Here's how the part is built. I have some questions about the finished solid (model axes, mm). Face numbers are marked on the shaded views. A direction names the side the tool comes from. Coordinates: 2 decimals unless noted, no trailing zeros. Write each loop counter-clockwise with the first axis right and the second up, starting at its lowest first coordinate (ties: lowest second). Pieces come first, ordered by that corner, then holes.
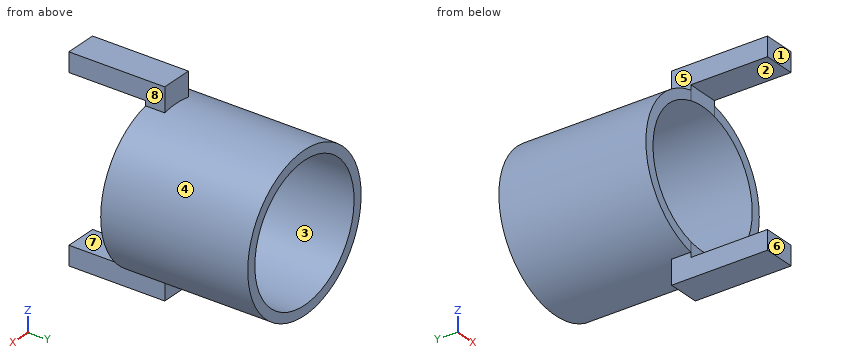
```python
from build123d import *

# Parameters (mm, degrees)
SKETCH1_W                = 5
SKETCH1_H                = 3
BOSS_EXTRUDE1_DEPTH      = 15
BOSS_EXTRUDE1_2_DEPTH    = 15
BOSS_EXTRUDE2_DEPTH      = 20
BOSS_EXTRUDE2_DEPTH_BACK = 3
SKETCH2_R                = 12
SKETCH4_W                = 5
SKETCH4_H                = 3.004832049
BOSS_EXTRUDE3_DEPTH      = 28
SKETCH3_R                = 10.5
CUT_EXTRUDE1_DEPTH       = 25


with BuildPart() as part:
    # Sketch1 → Boss-Extrude1 (new body)
    with BuildSketch(Plane(origin=(0, 0, 0), x_dir=(1, 0, 0), z_dir=(0, 1, 0))):
        with Locations((0, -14)):
            Rectangle(SKETCH1_W, SKETCH1_H)
    extrude(amount=BOSS_EXTRUDE1_DEPTH)



with BuildPart() as body_2:
    # Sketch1 → Boss-Extrude1 2 (new body)
    with BuildSketch(Plane(origin=(0, 0, 0), x_dir=(1, 0, 0), z_dir=(0, 1, 0))):
        with Locations((0, 14)):
            Rectangle(SKETCH1_W, SKETCH1_H)
    extrude(amount=BOSS_EXTRUDE1_2_DEPTH)


with BuildPart() as body_3:
    # Sketch2 → Boss-Extrude2 (new, two sides: drawn at the far end of the back side and taken through both)
    with BuildSketch(Plane(origin=(0, 15, 0), x_dir=(1, 0, 0), z_dir=(0, 1, 0)).offset(-BOSS_EXTRUDE2_DEPTH_BACK)):
        with Locations(Location((0, 0, 0), (0, 0, 270))):
            Circle(SKETCH2_R)
    extrude(amount=BOSS_EXTRUDE2_DEPTH + BOSS_EXTRUDE2_DEPTH_BACK)


with BuildPart() as part_1:
    add(part.part)

    add(body_2.part)  # Boss-Extrude3 merges body 2

    add(body_3.part)  # Boss-Extrude3 merges body 3
    # Sketch4 → Boss-Extrude3 (add)
    with BuildSketch(Plane.XY.offset(-12.5)):
        with Locations((0, 13.497583976)):
            Rectangle(SKETCH4_W, SKETCH4_H)
    extrude(amount=BOSS_EXTRUDE3_DEPTH)

    # Sketch3 → Cut-Extrude1 (cut)
    with BuildSketch(Plane(origin=(0, 35, 0), x_dir=(1, 0, 0), z_dir=(0, 1, 0))):
        with Locations(Location((0, 0, 0), (0, 0, 270))):
            Circle(SKETCH3_R)
    extrude(amount=-CUT_EXTRUDE1_DEPTH, mode=Mode.SUBTRACT)


solid = part_1.part
```
1) Imagine slicing it at D-D on y = 21.5. Please give me the cut outline in (x, z), then the cut area to 3 significant figures.
Values follow:
outline: circle Ø24 at (0, 0); hole circle Ø21 at (0, 0)
area: 106 mm2
2) Will these pins go through, and if not, where does the flat tip stop? pin 1 (10 mm diameter, centred on y = 4.5, z = 12, fed in from -X); pin 2 (10.5 mm diameter, centred on x = -6, z = 4.5, fed in from -Y); pin 3 (5 mm diameter, centred on y = 20, z = -10.5, fed in from +X); pin 4 (7.5 mm diameter, centred on x = 6, z = -1.5, fed in from -Y).
Values follow:
pin 1: stops at x = -2.5
pin 2: stops at y = 12
pin 3: stops at x = 8.94
pin 4: passes through
3) On a 3-axis mill with a long thin cutter (end or side, diameter ignored), from which of +Z, -Z, +X, -X, +Y, -Y can I reach the whole of each face in a straight line? I mean the marked faces 5, 6, 7 and 8. Say none if no direction works.
Values follow:
face 5: +Z, -X, +Y, -Y
face 6: +Z, -Z, +X, -X, -Y
face 7: +X, -X, -Y
face 8: +Z, +X, +Y, -Y
4) Imagine slicing it at C-C on x = 0. Please give me the cut outline in (y, z), then the cut area to 3 significant figures.
Values follow:
outline: (0, -15.5) - (15, -15.5) - (15, -12) - (35, -12) - (35, -10.5) - (12, -10.5) - (12, -12.5) - (0, -12.5) - close; (0, 12.5) - (12, 12.5) - (12, 10.5) - (35, 10.5) - (35, 12) - (15, 12) - (15, 15.5) - (0, 15.5) - close
area: 162 mm2
5) Imagine slicing it at B-B on z = 0. Please give me the cut outline in (x, y), then the cut area to 3 significant figures.
Values follow:
outline: (-12, 12) - (-10.5, 12) - (-10.5, 35) - (-12, 35) - close; (10.5, 12) - (12, 12) - (12, 35) - (10.5, 35) - close
area: 69.0 mm2
6) Imagine slicing it at A-A on y = 6. Please give me the cut outline in (x, z).
Values follow:
outline: (-2.5, -15.5) - (2.5, -15.5) - (2.5, -12.5) - (-2.5, -12.5) - close; (-2.5, 12.5) - (2.5, 12.5) - (2.5, 15.5) - (-2.5, 15.5) - close
7) We'd pull the mould along Z, two halves only. Please class the marked faces 1, 2, 3 and 4: pulls with the +Z half, pulls with the -Z half, needs draft (parallel to the pull), parting line crosses it, or undercut.
Values follow:
face 1: needs draft
face 2: undercut
face 3: undercut
face 4: parting line crosses it
8) I need wall thicknesses on probe 1 along X at (y, z) = (29, 0); probe 2 along Z at (x, y) = (1.75, 8.5); probe 3 along X at (y, z) = (27, -2.5). Which ranges of each line are inside material? Lowest first, please.
Values follow:
probe 1: x = -12 to -10.5, 10.5 to 12
probe 2: z = -15.5 to -12.5, 12.5 to 15.5
probe 3: x = -11.74 to -10.2, 10.2 to 11.74
